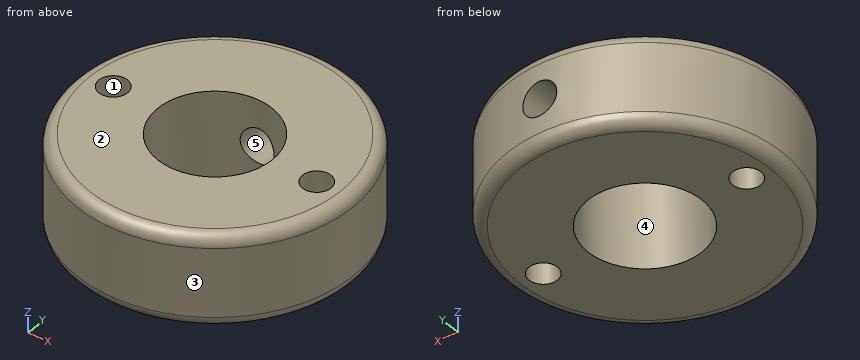
```python
from build123d import *

# Parameters (mm, degrees)
SKETCH1_W                  = 24
SKETCH1_H                  = 24
BOSS_EXTRUDE1_DEPTH        = 8
M3_TAPPED_HOLE1_D          = 2.5
F_10_0_10_DIAMETER_HOLE1_D = 10
F_3_0MM_DOWEL_HOLE1_REACH  = 30
F_3_0MM_DOWEL_HOLE1_BORE_R = 1.5
SKETCH15_R                 = 16.970562748
SKETCH15_R_2               = 12
CUT_EXTRUDE1_DEPTH         = 10
FILLET1_R                  = 1


with BuildPart() as part:
    # Sketch1 → Boss-Extrude1 (new body)
    with BuildSketch(Plane.XY):
        Rectangle(SKETCH1_W, SKETCH1_H)
    extrude(amount=BOSS_EXTRUDE1_DEPTH)

    # M3 Tapped Hole1 (through all)
    with Locations(Plane.XY.offset(8)):
        with Locations((9, 0), (-9, 0)):
            Hole(M3_TAPPED_HOLE1_D / 2)

    # Ø10.0 (10) Diameter Hole1 (through all)
    with Locations(Plane(origin=(0, 0, 0), x_dir=(-1, 0, 0), z_dir=(0, 0, -1))):
        with Locations((0, 0)):
            Hole(F_10_0_10_DIAMETER_HOLE1_D / 2)

    # Ø3.0mm Dowel Hole1 bore → Ø3.0mm Dowel Hole1 (cut, up to next)
    with BuildSketch(Plane(origin=(0, 12, 0), x_dir=(1, 0, 0), z_dir=(0, 1, 0)), mode=Mode.PRIVATE) as f_3_0mm_dowel_hole1_sk1:
        with Locations((0, -4)):
            Circle(F_3_0MM_DOWEL_HOLE1_BORE_R)
    f_3_0mm_dowel_hole1_tool1 = extrude(f_3_0mm_dowel_hole1_sk1.sketch, amount=-F_3_0MM_DOWEL_HOLE1_REACH, mode=Mode.PRIVATE) & part.part
    add(f_3_0mm_dowel_hole1_tool1.solids().sort_by_distance((0, 12, 4))[0], mode=Mode.SUBTRACT)

    # Sketch15 → Cut-Extrude1 (cut)
    with BuildSketch(Plane.XY.offset(8)):
        Circle(SKETCH15_R)
        Circle(SKETCH15_R_2, mode=Mode.SUBTRACT)
    extrude(amount=-CUT_EXTRUDE1_DEPTH, mode=Mode.SUBTRACT)

    # Fillet1
    fillet1_edges = [part.edges().sort_by_distance(p)[0] for p in [
        (-12, 0, 0),
        (-12, 0, 8),
    ]]
    fillet(fillet1_edges, radius=FILLET1_R)


solid = part.part
```
The model under review builds one solid part; all positions refer to its coordinate system, in mm. Face numbers are marked on the shaded views. A direction names the side the tool comes from. Coordinates: 2 decimals unless noted, no trailing zeros. Write each loop counter-clockwise with the first axis right and the second up, starting at its lowest first coordinate (ties: lowest second). Pieces come first, ordered by that corner, then holes. Notation, with made-up numbers: (57, 43) -> (70, 43) arc R16 cw to (70, 49) -> close; hole circle Ø1 at (-9, 48.5). An arc over 180 degrees is marked (long way). One line per item, written item: value. Start each with the question number.
Q1. The part is to be moulded in two halves that separate along Y. For the marked faces 1, 2 and 3, say which applies: +Y half, -Y half, draft (parallel to the pull), parting line (faces both ways), or undercut.
Q2. Add section B-B, the plane y = 0. Give the boundary of the cut face in (x, z), then the cut area to 3 significant figures.
Q3. Add section C-C, the plane z = 3. Give the boundary of the cut face in (x, y).
Q4. To check wall thickness, follow probe 1 along Z at (x, y) = (0, 7.25); probe 2 along Y at (x, z) = (0, 2); probe 3 along Y at (x, z) = (9, 5.5). State the ranges of each line that lie inside material, in increasing order.
Q5. Add section D-D, the plane z = 4.75. Give the boundary of the cut face in (x, y), then the cut area to 3 significant figures.
Q6. Add section A-A, the plane x = 0. Give the boundary of the cut face in (y, z), then the cut area to 3 significant figures.
Q7. For the marked faces 4 and 5, list the 3-axis set-ups (+Z, -Z, +X, -X, +Y, -Y) from which the entire face can be reached by the end or side of a thin tool; tool diameter is ignored.
Q8. Clearance check with flat-ended pins moving along their axes: P1, Ø4, axis at x = -7, z = 7, coming from the -Y side; P2, Ø1.5, axis at y = -4.5, z = 4.5, coming from the -X side; P3, Ø6, axis at x = 4, y = -5.5, coming from the -Z side; P4, Ø2, axis at x = 5, z = 4, coming from the +Y side. State where each tip first meets the part, or that it passes through.
Response:
1. face 1: undercut
1. face 2: draft
1. face 3: parting line
2. outline: (-12, 1) arc R1 ccw to (-11, 0) -> (-10.25, 0) -> (-10.25, 8) -> (-11, 8) arc R1 ccw to (-12, 7) -> close; (-7.75, 0) -> (-5, 0) -> (-5, 8) -> (-7.75, 8) -> close; (5, 0) -> (7.75, 0) -> (7.75, 8) -> (5, 8) -> close; (10.25, 0) -> (11, 0) arc R1 ccw to (12, 1) -> (12, 7) arc R1 ccw to (11, 8) -> (10.25, 8) -> close
2. area: 71.1 mm²
3. outline: (-1.12, 4.87) -> (-1.12, 11.95) arc R12 ccw (long way) to (1.12, 11.95) -> (1.12, 4.87) arc R5 cw (long way) to start; hole circle Ø2.5 at (-9, 0); hole circle Ø2.5 at (9, 0)
4. probe 1: 0 to 2.5, 5.5 to 8
4. probe 2: -12 to -5, 5 to 12
4. probe 3: -7.94 to -1.25, 1.25 to 7.94
5. outline: (-1.3, 4.83) -> (-1.3, 11.93) arc R12 ccw (long way) to (1.3, 11.93) -> (1.3, 4.83) arc R5 cw (long way) to start; hole circle Ø2.5 at (-9, 0); hole circle Ø2.5 at (9, 0)
5. area: 346 mm²
6. outline: (-12, 1) arc R1 ccw to (-11, 0) -> (-5, 0) -> (-5, 8) -> (-11, 8) arc R1 ccw to (-12, 7) -> close; (5, 0) -> (11, 0) arc R1 ccw to (12, 1) -> (12, 2.5) -> (5, 2.5) -> close; (5, 5.5) -> (12, 5.5) -> (12, 7) arc R1 ccw to (11, 8) -> (5, 8) -> close
6. area: 90.1 mm²
7. face 4: +Z, -Z
7. face 5: +Y
8. P1: y = -10.91
8. P2: x = -11.4
8. P3: z = 0
8. P4: y = 11.31
